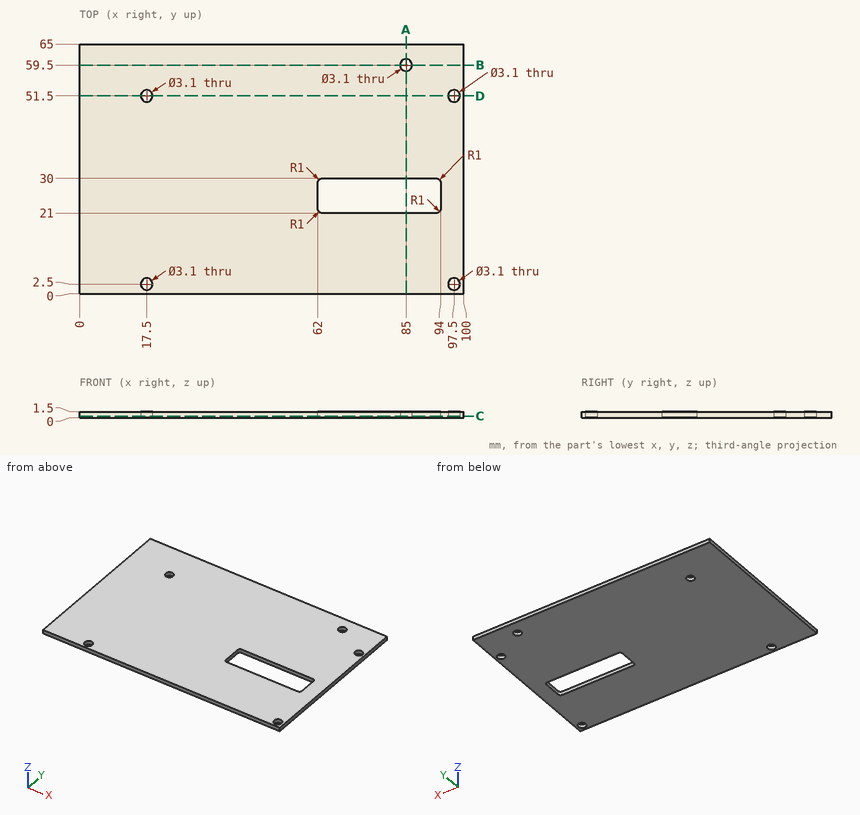
Design review of the part shown in the three views and the two pictorial views. Dimensions are in mm from the part's minimum x, y and z. Give positions to 0.01 mm unless a question says otherwise; leave off trailing zeros. Write each loop counter-clockwise with the first axis right and the second up, starting at its lowest first coordinate (ties: lowest second). Pieces come first, ordered by that corner, then holes. Notation, with made-up numbers: M 59.5,5.25 L 92.5,5.25 A18 ccw 92.5,22.25 Z; hole C 38,33.25 d6. An arc over 180 degrees is marked long. Answer in a Markdown table with one row per item.
Item 1: Add section A-A on x = 85. Give the boundary of the cut face in (y, z).
Check sheet entries:
| item | result |
|---|---|
| outline | M 0,0 L 21,0 L 21,1.5 L 0,1.5 Z; M 30,0 L 57.95,0 L 57.95,1.5 L 30,1.5 Z; M 61.05,0 L 65,0 L 65,1.5 L 61.05,1.5 Z |
Item 2: For line 1 along Y through (x, z) = (97.5, 0.5); line 2 along X through (y, z) = (29, 1.25); line 3 along Y through (x, z) = (91, 0.7), list the stretches that pass through material, from the lowest coordinate up.
Check sheet entries:
| item | result |
|---|---|
| line 1 | 0 to 0.95, 4.05 to 49.95, 53.05 to 65 |
| line 2 | 0 to 62, 94 to 100 |
| line 3 | 0 to 21, 30 to 65 |
Item 3: Add section B-B on y = 59.5. Give the boundary of the cut face in (x, z), plus the area to 3 significant figures.
Check sheet entries:
| item | result |
|---|---|
| outline | M 0,0 L 83.45,0 L 83.45,1.5 L 0,1.5 Z; M 86.55,0 L 100,0 L 100,1.5 L 86.55,1.5 Z |
| area | 145 mm2 |
Item 4: Add section D-D on y = 51.5. Give the boundary of the cut face in (x, z).
Check sheet entries:
| item | result |
|---|---|
| outline | M 0,0 L 15.95,0 L 15.95,1.5 L 0,1.5 Z; M 19.05,0 L 95.95,0 L 95.95,1.5 L 19.05,1.5 Z; M 99.05,0 L 100,0 L 100,1.5 L 99.05,1.5 Z |
Item 5: Add section C-C on z = 0.35. Give the boundary of the cut face in (x, y), plus the area to 3 significant figures.
Check sheet entries:
| item | result |
|---|---|
| outline | M 0,0 L 100,0 L 100,65 L 0,65 Z; hole C 17.5,2.5 d3.1; hole C 17.5,51.5 d3.1; hole M 62,22 A1 ccw 63,21 L 93,21 A1 ccw 94,22 L 94,29 A1 ccw 93,30 L 63,30 A1 ccw 62,29 Z; hole C 85,59.5 d3.1; hole C 97.5,2.5 d3.1; hole C 97.5,51.5 d3.1 |
| area | 6,180 mm2 |
